Can you work these out from the model? Positions are in its coordinate system, mm. Face numbers are marked on the shaded views. A direction names the side the tool comes from. Coordinates: 2 decimals unless noted, no trailing zeros. Loops run counter-clockwise (first coordinate to the right, second up) from the corner with the lowest first, then second, coordinate; pieces in that order, holes last.
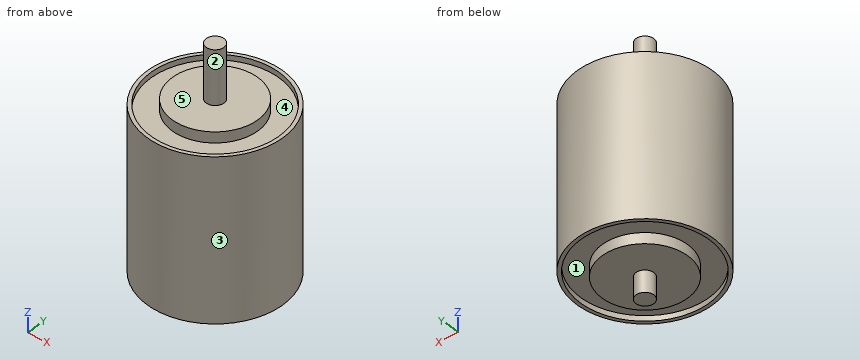
```python
from build123d import *

# Parameters (mm, degrees)
SKETCH7_R           = 120
BOSS_EXTRUDE1_DEPTH = 30
SKETCH8_R           = 25
BOSS_EXTRUDE2_DEPTH = 60
BOSS_EXTRUDE3_START = 150
SKETCH11_R          = 25
BOSS_EXTRUDE3_DEPTH = 150


# Read off the part's stored shape, not the designer's step: Revolve-Thin1
with BuildPart() as part:
    # Revolve-Thin1 outline → Revolve-Thin1 (revolve)
    with BuildSketch(Plane.XZ.offset(190)):
        Polygon((180, 309.593023256), (0, 309.593023256), (0, 299.593023256), (180, 299.593023256), (180, -100.406976744), (0, -100.406976744), (0, -110.406976744), (180, -110.406976744), (180, -125.406976744), (190, -125.406976744), (190, 324.593023256), (180, 324.593023256), align=None)
    revolve(axis=Axis((0, -190, 0), (0, 0, 1)))

    # Sketch7 → Boss-Extrude1 (add)
    with BuildSketch(Plane(origin=(0, 0, -110.406976744), x_dir=(-1, 0, 0), z_dir=(0, 0, -1))):
        with Locations(Location((0, -190, 0), (0, 0, 90))):
            Circle(SKETCH7_R)
    boss_extrude1 = extrude(amount=BOSS_EXTRUDE1_DEPTH)

    # Mirror1: Boss-Extrude1 across plane
    add(boss_extrude1.mirror(Plane(origin=(0, 0, 99.593023256), x_dir=(1, 0, 0), z_dir=(0, 0, -1))))

    # Sketch8 → Boss-Extrude2 (add)
    with BuildSketch(Plane(origin=(0, 0, -140.406976744), x_dir=(-1, 0, 0), z_dir=(0, 0, -1))):
        with Locations(Location((0, -190, 0), (0, 0, 90))):
            Circle(SKETCH8_R)
    extrude(amount=BOSS_EXTRUDE2_DEPTH)

    # Sketch11 → Boss-Extrude3 (add)
    with BuildSketch(Plane.XY.offset(339.593023256).offset(BOSS_EXTRUDE3_START)):
        with Locations(Location((0, -190, 0), (0, 0, 90))):
            Circle(SKETCH11_R)
    extrude(amount=-BOSS_EXTRUDE3_DEPTH)


solid = part.part
```
(1) I want a section at D-D on y = -85.5. Write out the boundary of the cut face in (x, z).
Check values:
outline: (-158.68, -125.41) - (-146.56, -125.41) - (-146.56, -110.41) - (-58.99, -110.41) - (-58.99, -140.41) - (58.99, -140.41) - (58.99, -110.41) - (146.56, -110.41) - (146.56, -125.41) - (158.68, -125.41) - (158.68, 324.59) - (146.56, 324.59) - (146.56, 309.59) - (58.99, 309.59) - (58.99, 339.59) - (-58.99, 339.59) - (-58.99, 309.59) - (-146.56, 309.59) - (-146.56, 324.59) - (-158.68, 324.59) - close; hole (-146.56, -100.41) - (146.56, -100.41) - (146.56, 299.59) - (-146.56, 299.59) - close
(2) I'm going to push flat-ended pins straight in: pin 1 (8 mm diameter, centred on y = -55, z = 73, fed in from -X); pin 2 (5 mm diameter, centred on x = 49, y = -228, fed in from -Z); pin 3 (1 mm diameter, centred on y = -223, z = 339, fed in from +X). Where does each tip first touch, or does it pass through?
Check values:
pin 1: stops at x = -137.62
pin 2: stops at z = -140.41
pin 3: stops at x = 115.52
(3) If we mould it in two halves opening along X, with no side actions, what happens to the marked faces 3, 4 and 5? For each: released by +X, released by -X, zero draft, split by the parting line, or undercut.
Check values:
face 3: split by the parting line
face 4: undercut
face 5: zero draft
(4) I want a section at B-B on x = -99. Write out the boundary of the cut face in (y, z).
Check values:
outline: (-352.17, -125.41) - (-340.33, -125.41) - (-340.33, -110.41) - (-257.82, -110.41) - (-257.82, -140.41) - (-122.18, -140.41) - (-122.18, -110.41) - (-39.67, -110.41) - (-39.67, -125.41) - (-27.83, -125.41) - (-27.83, 324.59) - (-39.67, 324.59) - (-39.67, 309.59) - (-122.18, 309.59) - (-122.18, 339.59) - (-257.82, 339.59) - (-257.82, 309.59) - (-340.33, 309.59) - (-340.33, 324.59) - (-352.17, 324.59) - close; hole (-340.33, -100.41) - (-39.67, -100.41) - (-39.67, 299.59) - (-340.33, 299.59) - close
(5) I want a section at C-C on z = 203. Write out the boundary of the cut face in (x, y).
Check values:
outline: circle Ø380 at (0, -190); hole circle Ø360 at (0, -190)
(6) If I drill on probe 1 along Z at (x, y) = (-128.5, -174); probe 2 along Z at (x, y) = (47.5, -115); probe 3 along Y at (x, z) = (105.5, -122.5), over which ranges is the centre line in solid material (lowest first)?
Check values:
probe 1: z = -110.41 to -100.41, 299.59 to 309.59
probe 2: z = -140.41 to -100.41, 299.59 to 339.59
probe 3: y = -348.02 to -335.84, -247.18 to -132.82, -44.16 to -31.98
(7) Which directions (+Z, -Z, +X, -X, +Y, -Y) give clear straight access to the entire face, cutting with the end or side of a thin tool? Please do the marked faces 1 and 2.
Check values:
face 1: -Z
face 2: +Z
